from build123d import *

# Parameters (mm, degrees)
F0_W     = 140
F0_H     = 50
F1_DEPTH = 8
F2_SIZE  = 2.5
F4_D     = 3.5
F5_D     = 6.5
F6_D     = 11


with BuildPart() as f1:
    # F0 (on Front) → F1 (new body)
    with BuildSketch(Plane.XZ):
        Rectangle(F0_W, F0_H)
    extrude(amount=F1_DEPTH)

    # F2
    f2_edges = [f1.edges().sort_by_distance(p)[0] for p in [
        (70, -4, 25),
        (-70, -4, 25),
        (70, -4, -25),
        (-70, -4, -25),
    ]]
    chamfer(f2_edges, length=F2_SIZE)

    # F4 (through all)
    with Locations(Plane.XZ.offset(8)):
        with Locations((62.5, 17.5), (62.5, -17.5), (-62.5, -17.5), (-62.5, 17.5)):
            Hole(F4_D / 2)

    # F5 (through all)
    with Locations(Plane.XZ.offset(8)):
        with Locations((42, 15), (-42, 15)):
            Hole(F5_D / 2)

    # F6 (through all)
    with Locations(Plane.XZ.offset(8)):
        with Locations((0, 0)):
            Hole(F6_D / 2)


solid = f1.part
Read the model definition and answer for the solid it produces. Units are mm, in the model's axes. Coordinates: 2 decimals unless noted, no trailing zeros. Loops run counter-clockwise (first coordinate to the right, second up) from the corner with the lowest first, then second, coordinate; pieces in that order, holes last. Notation, with made-up numbers: (67.25, 76.25) -> (126.25, 76.25) arc R17 cw to (126.25, 97.25) -> close; hole circle Ø3 at (21.5, -1.5). An arc over 180 degrees is marked (long way). Write item = value, one per line. Start each with the question number.
1) The part is cut by section C-C, the plane x = 42. Determine the outline of the cut face in (y, z).
2) Find the intervals of material crossed by L1, parallel to Z at x = -62.5, y = -5.5; L2, parallel to Z at x = -42, y = -3; L3, parallel to Z at x = 0, y = -2.25, in increasing order. Write a range as from..to.
3) The part is cut by section A-A, the plane x = 62.5. Determine the outline of the cut face in (y, z), plus the area to 3 significant figures.
4) Given P1, Ø3, axis at x = -62.5, z = 17.5, coming from the -Y side, flat-ended and moving along its own axis, determine where the tip first touches the part or whether it passes through.
5) The mould has two halves that part along Z. Classify faces 1 (the face through (1.19, -3.94, -5.37)), 2 (the face through (-68.7, -3.9, -23.8)), 3 (the face through (-70, -4, 0)): pulls with the +Z half, pulls with the -Z half, needs draft (parallel to the pull), parting line crosses it, or undercut.
6) The part is cut by section D-D, the plane y = -2.25. Determine the outline of the cut face in (x, z).
7) The part is cut by section B-B, the plane z = -17.5. Determine the outline of the cut face in (x, y).
Result:
q1.outline = (-8, -25) -> (0, -25) -> (0, 11.75) -> (-8, 11.75) -> close; (-8, 18.25) -> (0, 18.25) -> (0, 25) -> (-8, 25) -> close
q2.L1 = -25..-19.25, -15.75..15.75, 19.25..25
q2.L2 = -25..11.75, 18.25..25
q2.L3 = -25..-5.5, 5.5..25
q3.outline = (-8, -25) -> (0, -25) -> (0, -19.25) -> (-8, -19.25) -> close; (-8, -15.75) -> (0, -15.75) -> (0, 15.75) -> (-8, 15.75) -> close; (-8, 19.25) -> (0, 19.25) -> (0, 25) -> (-8, 25) -> close
q3.area = 344 mm²
q4.P1 = through
q5.face_1 = undercut
q5.face_2 = pulls with the -Z half
q5.face_3 = needs draft
q6.outline = (-70, -22.5) -> (-67.5, -25) -> (67.5, -25) -> (70, -22.5) -> (70, 22.5) -> (67.5, 25) -> (-67.5, 25) -> (-70, 22.5) -> close; hole circle Ø3.5 at (-62.5, -17.5); hole circle Ø3.5 at (-62.5, 17.5); hole circle Ø6.5 at (-42, 15); hole circle Ø11 at (0, 0); hole circle Ø6.5 at (42, 15); hole circle Ø3.5 at (62.5, -17.5); hole circle Ø3.5 at (62.5, 17.5)
q7.outline = (-70, -8) -> (-64.25, -8) -> (-64.25, 0) -> (-70, 0) -> close; (-60.75, -8) -> (60.75, -8) -> (60.75, 0) -> (-60.75, 0) -> close; (64.25, -8) -> (70, -8) -> (70, 0) -> (64.25, 0) -> close
